Source: three-view drawing plus pictorial views. Frame: mm from the lowest corner of the part. A direction names the side the tool comes from. Give positions to 0.01 mm unless a question says otherwise; leave off trailing zeros. Order: outer loops, then holes, each group sorted by start corner. A loop starts at its lowest first (then second) coordinate and runs counter-clockwise, first axis right, second up. Notation, with made-up numbers: (89.25, -20) - (133.25, -20) arc R15 ccw to (133.25, -4) - close; hole circle Ø9 at (77, 34). An arc over 180 degrees is marked (long way). Answer in a Markdown table with one row per item. Add a question column.
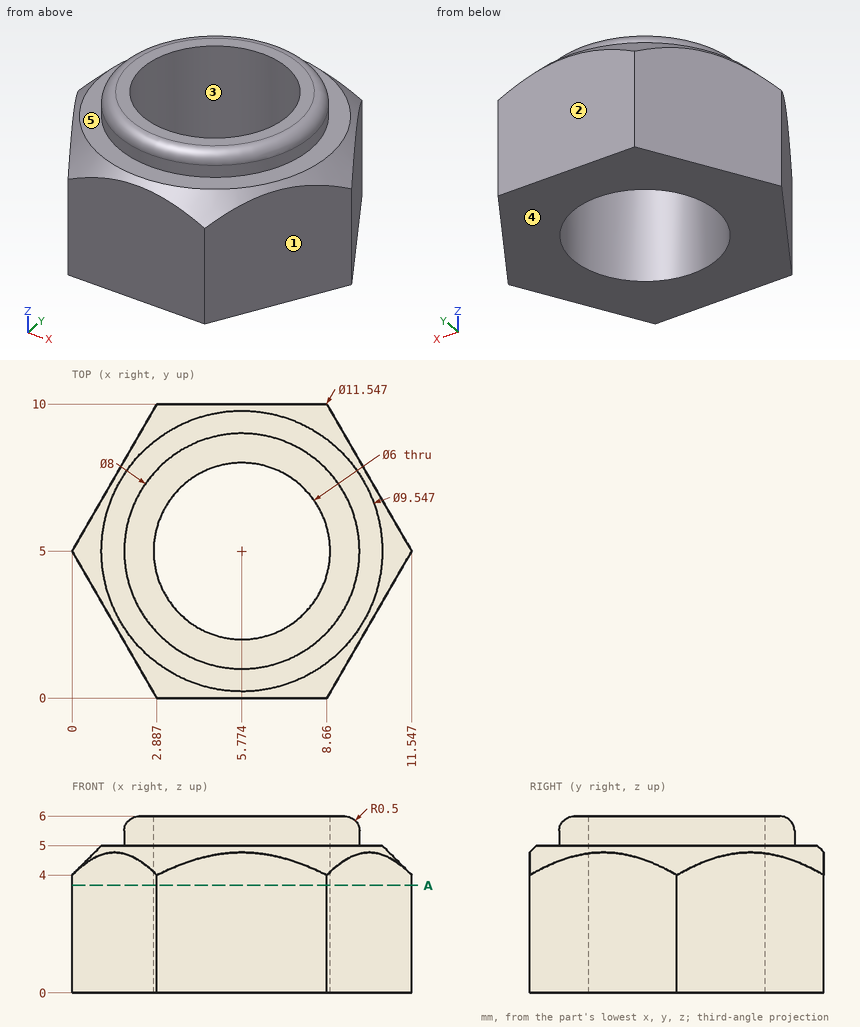
Q1. Line query: probe 1 along Z at (x, y) = (1.75, 5.25); probe 2 along Y at (x, z) = (6, 2); probe 3 along Y at (x, z) = (4.5, 4.85) (1 decimal). Output: solid intervals per line, ascending.
Q2. Section A-A, the plane z = 3.65. Return loops of the section in (x, y).
Q3. Contact query for a flat-ended pin moving along its axis: P1, Ø3, axis at y = 5, z = 1.5, coming from the -X side. Output: stop coordinate, or through.
Q4. Pull-direction query (Y, two-part tool) for the marked faces 1, 2 and 3; classes: +Y half, -Y half, draft (parallel to the pull), parting line (faces both ways), or undercut.
Q5. Access query for the marked faces 4 and 5. Directions: +Z, -Z, +X, -X, +Y, -Y. A direction counts if a zero-diameter tool reaches every point of the face in a straight line with its end or side. Return the directions, or none.
Computed:
| question | item | result |
|---|---|---|
| 1 | probe 1 | z = 0 to 5 |
| 1 | probe 2 | y = 0 to 2.01, 7.99 to 10 |
| 1 | probe 3 | y = 0.2 to 2.3, 7.7 to 9.8 |
| 2 | outline | (0, 5) - (2.89, 0) - (8.66, 0) - (11.55, 5) - (8.66, 10) - (2.89, 10) - close; hole circle Ø6 at (5.77, 5) |
| 3 | P1 | stops at x = 0 |
| 4 | face 1 | -Y half |
| 4 | face 2 | +Y half |
| 4 | face 3 | undercut |
| 5 | face 4 | -Z, +X, -X, +Y, -Y |
| 5 | face 5 | +Z |
